The model under review builds one solid part; all positions refer to its coordinate system, in mm. Give positions to 0.01 mm unless a question says otherwise; leave off trailing zeros. Loops run counter-clockwise (first coordinate to the right, second up) from the corner with the lowest first, then second, coordinate; pieces in that order, holes last. Notation, with made-up numbers: M 77.25,58.25 L 99.25,58.25 A11 ccw 99.25,64.25 Z; hole C 9,52.5 d3. An arc over 180 degrees is marked long. One line per item, written item: value. Start each with the question number.
Q1. We need section C-C on x = 37. Give the number of separate pieces and of enclosed holes in the cut face, plus the area to 3 significant figures.
Q2. Mouldability with a two-part tool opening along Y and no side actions: class faces 1 (the face through (-0.867, -3.905, 0.986)), 2 (the face through (24, 15, 18)), 3 (the face through (-0.7, 16, 20.1)) as released by +Y, released by -Y, zero draft, split by the parting line, or undercut.
Q3. For pin 1 (5 mm diameter, centred on x = -24, y = 0, fed in from +Z), flat-tipped, find the tip position at first contact; note if it passes through.
Q4. To check wall thickness, follow line 1 along Y through (x, z) = (2.5, 25.5); line 2 along Z through (x, y) = (-3.5, 5.5); line 3 along Z through (x, y) = (16, 15.2). State the ranges of each line that lie inside material, in increasing order. Write a range as from..to.
Q5. We need section A-A on z = 28.5. Write out the cut boundary in (x, y), plus the area to 3 significant figures.
Q6. We need section B-B on x = 7.5. Write out the cut boundary in (y, z).
```python
from build123d import *

# Parameters (mm, degrees)
F0_W     = 96
F0_H     = 32
F0_R     = 2
F0_R_2   = 1.5
F0_R_3   = 4
F5_DEPTH = 2
F3_W     = 96
F3_H     = 32
F3_R     = 2
F3_R_2   = 1.5
F3_R_3   = 4
F6_DEPTH = 2
F4_W     = 96
F4_H     = 32
F4_R     = 2
F4_R_2   = 1.5
F4_R_3   = 4
F7_DEPTH = 2
F8_R     = 2


with BuildPart() as f5:
    # F0 (on Top) → F5 (new body)
    with BuildSketch(Plane.XY):
        Rectangle(F0_W, F0_H)
        with Locations((-37.656854, -5.656854)):
            Circle(F0_R, mode=Mode.SUBTRACT)
        with Locations((-32, -8)):
            Circle(F0_R, mode=Mode.SUBTRACT)
        with Locations((-26.343146, -5.656854)):
            Circle(F0_R, mode=Mode.SUBTRACT)
        with Locations((0, -7.5)):
            Circle(F0_R_2, mode=Mode.SUBTRACT)
        with Locations((32, -8)):
            Circle(F0_R, mode=Mode.SUBTRACT)
        with Locations((26.343146, -5.656854)):
            Circle(F0_R, mode=Mode.SUBTRACT)
        with Locations((37.656854, -5.656854)):
            Circle(F0_R, mode=Mode.SUBTRACT)
        with BuildLine():
            ThreePointArc((-42, 0), (-40, 2), (-38, 0))
            ThreePointArc((-38, 0), (-40, -2), (-42, 0))
        make_face(mode=Mode.SUBTRACT)
        with BuildLine():
            ThreePointArc((-28, 0), (-32, -4), (-36, 0))
            ThreePointArc((-36, 0), (-32, 4), (-28, 0))
        make_face(mode=Mode.SUBTRACT)
        with Locations((-37.656854, 5.656854)):
            Circle(F0_R, mode=Mode.SUBTRACT)
        with Locations((-26.343146, 5.656854)):
            Circle(F0_R, mode=Mode.SUBTRACT)
        with Locations((-24, 0)):
            Circle(F0_R, mode=Mode.SUBTRACT)
        with Locations((-16, 0)):
            Circle(F0_R_3, mode=Mode.SUBTRACT)
        with Locations((-7.5, 0)):
            Circle(F0_R_2, mode=Mode.SUBTRACT)
        with Locations((-32, 8)):
            Circle(F0_R, mode=Mode.SUBTRACT)
        Circle(F0_R_3, mode=Mode.SUBTRACT)
        with Locations((7.5, 0)):
            Circle(F0_R_2, mode=Mode.SUBTRACT)
        with Locations((16, 0)):
            Circle(F0_R_3, mode=Mode.SUBTRACT)
        with Locations((0, 7.5)):
            Circle(F0_R_2, mode=Mode.SUBTRACT)
        with Locations((24, 0)):
            Circle(F0_R, mode=Mode.SUBTRACT)
        with Locations((32, 0)):
            Circle(F0_R_3, mode=Mode.SUBTRACT)
        with Locations((40, 0)):
            Circle(F0_R, mode=Mode.SUBTRACT)
        with Locations((26.343146, 5.656854)):
            Circle(F0_R, mode=Mode.SUBTRACT)
        with Locations((37.656854, 5.656854)):
            Circle(F0_R, mode=Mode.SUBTRACT)
        with Locations((32, 8)):
            Circle(F0_R, mode=Mode.SUBTRACT)
    extrude(amount=F5_DEPTH)

    # F3 (on face) → F6 (join)
    with BuildSketch(Plane(origin=(0, 16, 0), x_dir=(-1, 0, 0), z_dir=(0, 1, 0))):
        with Locations((0, 16)):
            Rectangle(F3_W, F3_H)
        with Locations((-37.656854, 10.343146)):
            Circle(F3_R, mode=Mode.SUBTRACT)
        with Locations((-32, 8)):
            Circle(F3_R, mode=Mode.SUBTRACT)
        with Locations((-26.343146, 10.343146)):
            Circle(F3_R, mode=Mode.SUBTRACT)
        with Locations((0, 8.5)):
            Circle(F3_R_2, mode=Mode.SUBTRACT)
        with Locations((32, 8)):
            Circle(F3_R, mode=Mode.SUBTRACT)
        with Locations((26.343146, 10.343146)):
            Circle(F3_R, mode=Mode.SUBTRACT)
        with Locations((37.656854, 10.343146)):
            Circle(F3_R, mode=Mode.SUBTRACT)
        with BuildLine():
            ThreePointArc((-42, 16), (-40, 18), (-38, 16))
            ThreePointArc((-38, 16), (-40, 14), (-42, 16))
        make_face(mode=Mode.SUBTRACT)
        with BuildLine():
            ThreePointArc((-28, 16), (-32, 12), (-36, 16))
            ThreePointArc((-36, 16), (-32, 20), (-28, 16))
        make_face(mode=Mode.SUBTRACT)
        with Locations((-37.656854, 21.656854)):
            Circle(F3_R, mode=Mode.SUBTRACT)
        with Locations((-26.343146, 21.656854)):
            Circle(F3_R, mode=Mode.SUBTRACT)
        with Locations((-24, 16)):
            Circle(F3_R, mode=Mode.SUBTRACT)
        with Locations((-16, 16)):
            Circle(F3_R_3, mode=Mode.SUBTRACT)
        with Locations((-7.5, 16)):
            Circle(F3_R_2, mode=Mode.SUBTRACT)
        with Locations((-32, 24)):
            Circle(F3_R, mode=Mode.SUBTRACT)
        with Locations((0, 16)):
            Circle(F3_R_3, mode=Mode.SUBTRACT)
        with Locations((7.5, 16)):
            Circle(F3_R_2, mode=Mode.SUBTRACT)
        with Locations((16, 16)):
            Circle(F3_R_3, mode=Mode.SUBTRACT)
        with Locations((0, 23.5)):
            Circle(F3_R_2, mode=Mode.SUBTRACT)
        with Locations((24, 16)):
            Circle(F3_R, mode=Mode.SUBTRACT)
        with Locations((32, 16)):
            Circle(F3_R_3, mode=Mode.SUBTRACT)
        with Locations((40, 16)):
            Circle(F3_R, mode=Mode.SUBTRACT)
        with Locations((26.343146, 21.656854)):
            Circle(F3_R, mode=Mode.SUBTRACT)
        with Locations((37.656854, 21.656854)):
            Circle(F3_R, mode=Mode.SUBTRACT)
        with Locations((32, 24)):
            Circle(F3_R, mode=Mode.SUBTRACT)
    extrude(amount=-F6_DEPTH)

    # F4 (on face) → F7 (join)
    with BuildSketch(Plane(origin=(0, -16, 0), x_dir=(-1, 0, 0), z_dir=(0, 1, 0))):
        with Locations((0, 16)):
            Rectangle(F4_W, F4_H)
        with Locations((-37.656854, 10.343146)):
            Circle(F4_R, mode=Mode.SUBTRACT)
        with Locations((-32, 8)):
            Circle(F4_R, mode=Mode.SUBTRACT)
        with Locations((-26.343146, 10.343146)):
            Circle(F4_R, mode=Mode.SUBTRACT)
        with Locations((0, 8.5)):
            Circle(F4_R_2, mode=Mode.SUBTRACT)
        with Locations((32, 8)):
            Circle(F4_R, mode=Mode.SUBTRACT)
        with Locations((26.343146, 10.343146)):
            Circle(F4_R, mode=Mode.SUBTRACT)
        with Locations((37.656854, 10.343146)):
            Circle(F4_R, mode=Mode.SUBTRACT)
        with Locations((-40, 16)):
            Circle(F4_R, mode=Mode.SUBTRACT)
        with BuildLine():
            ThreePointArc((-28, 16), (-32, 12), (-36, 16))
            ThreePointArc((-36, 16), (-32, 20), (-28, 16))
        make_face(mode=Mode.SUBTRACT)
        with Locations((-37.656854, 21.656854)):
            Circle(F4_R, mode=Mode.SUBTRACT)
        with Locations((-26.343146, 21.656854)):
            Circle(F4_R, mode=Mode.SUBTRACT)
        with Locations((-24, 16)):
            Circle(F4_R, mode=Mode.SUBTRACT)
        with Locations((-16, 16)):
            Circle(F4_R_3, mode=Mode.SUBTRACT)
        with Locations((-7.5, 16)):
            Circle(F4_R_2, mode=Mode.SUBTRACT)
        with Locations((-32, 24)):
            Circle(F4_R, mode=Mode.SUBTRACT)
        with Locations((0, 16)):
            Circle(F4_R_3, mode=Mode.SUBTRACT)
        with Locations((7.5, 16)):
            Circle(F4_R_2, mode=Mode.SUBTRACT)
        with Locations((16, 16)):
            Circle(F4_R_3, mode=Mode.SUBTRACT)
        with Locations((0, 23.5)):
            Circle(F4_R_2, mode=Mode.SUBTRACT)
        with Locations((24, 16)):
            Circle(F4_R, mode=Mode.SUBTRACT)
        with Locations((32, 16)):
            Circle(F4_R_3, mode=Mode.SUBTRACT)
        with Locations((40, 16)):
            Circle(F4_R, mode=Mode.SUBTRACT)
        with Locations((26.343146, 21.656854)):
            Circle(F4_R, mode=Mode.SUBTRACT)
        with Locations((37.656854, 21.656854)):
            Circle(F4_R, mode=Mode.SUBTRACT)
        with Locations((32, 24)):
            Circle(F4_R, mode=Mode.SUBTRACT)
    extrude(amount=F7_DEPTH)

    # F8
    f8_edges = [f5.edges().sort_by_distance(p)[0] for p in [
        (0, 16, 0),
        (48, 15, 32),
        (48, -15, 32),
        (0, -16, 0),
        (-48, 15, 32),
        (-48, -15, 32),
    ]]
    fillet(f8_edges, radius=F8_R)


solid = f5.part
```
Solved:
1. separate pieces: 7
1. enclosed holes: 0
1. area: 137 mm2
2. face 1: undercut
2. face 2: zero draft
2. face 3: released by +Y
3. pin 1: z = 2
4. line 1: -16..-14, 14..16
4. line 2: 0..2
4. line 3: 0.4..12, 20..32
5. outline: M -48,-16 L 48,-16 L 48,-14 L -48,-14 Z; M -48,14 L 48,14 L 48,16 L -48,16 Z
5. area: 384 mm2
6. outline: M -16,2 A2 ccw -14,0 L -1.5,0 L -1.5,2 L -14,2 L -14,14.5 L -16,14.5 Z; M -16,17.5 L -14,17.5 L -14,32 L -16,32 Z; M 1.5,0 L 14,0 A2 ccw 16,2 L 16,14.5 L 14,14.5 L 14,2 L 1.5,2 Z; M 14,17.5 L 16,17.5 L 16,32 L 14,32 Z
